Input: part model. Units: mm. Frame: model coordinates. Give positions to 0.01 mm unless a question says otherwise; leave off trailing zeros. Loops run counter-clockwise (first coordinate to the right, second up) from the corner with the lowest first, then second, coordinate; pieces in that order, holes last. Notation, with made-up numbers: (11.25, 80) -> (39.25, 80) arc R33 ccw to (39.25, 113) -> close; hole circle Ø5 at (0, 73). An arc over 180 degrees is marked (long way). Answer as a JSON object with one key per item and string values.
```python
from build123d import *

# Parameters (mm, degrees)
SKETCH_W        = 40
SKETCH_H        = 20
PAD_DEPTH       = 0.8
SKETCH001_R     = 1.7
POCKET_DEPTH    = 90.258029
SKETCH002_W     = 12.04
SKETCH002_H     = 10.6
POCKET001_DEPTH = 0.801


with BuildPart() as part:
    # Sketch → Pad (new body)
    with BuildSketch(Plane.XZ):
        Rectangle(SKETCH_W, SKETCH_H)
    extrude(amount=PAD_DEPTH)

    # Sketch001 (on Face6 of Pad) → Pocket (cut, through all)
    with BuildSketch(Plane.XZ.offset(0.8)):
        with Locations((-15.25, 0)):
            Circle(SKETCH001_R)
    pocket = extrude(amount=-POCKET_DEPTH, mode=Mode.SUBTRACT)

    # Mirrored: Pocket across YZ
    add(pocket.mirror(Plane.YZ), mode=Mode.SUBTRACT)

    # Sketch002 (on Face5 of Mirrored) → Pocket001 (cut, through all)
    with BuildSketch(Plane.XZ.offset(0.8)):
        with Locations((0, 1.445)):
            Rectangle(SKETCH002_W, SKETCH002_H)
    extrude(amount=-POCKET001_DEPTH, mode=Mode.SUBTRACT)


solid = part.part
```
Q1. Ray query, line 1 along Z through (x, y) = (15.25, -0.5); line 2 along Z through (x, y) = (-2, -0.45) (3 decimals); line 3 along X through (y, z) = (-0.55, -2.5). Return the intervals inside material, ascending.
Evaluation:
{"line 1": "z = -10 to -1.7, 1.7 to 10", "line 2": "z = -10 to -3.855, 6.745 to 10", "line 3": "x = -20 to -6.02, 6.02 to 20"}
Q2. Section C-C, the plane x = 2.5. Return the cut outline in (y, z) (3 decimals), then the cut area to 3 significant figures.
Evaluation:
{"outline": "(-0.8, -10) -> (0, -10) -> (0, -3.855) -> (-0.8, -3.855) -> close; (-0.8, 6.745) -> (0, 6.745) -> (0, 10) -> (-0.8, 10) -> close", "area": "7.52 mm2"}
Q3. Draft query along Z for faces 1 (the cylindrical face through (13.63, -0.41, 0.51)), 2 (the flat face through (-0.3, -0.8, -4.3)). Return one class per face: +Z half, -Z half, draft (parallel to the pull), parting line (faces both ways), or undercut.
Evaluation:
{"face 1": "undercut", "face 2": "draft"}
Q4. Pin query (flat end, axial travel): pin 1 (5 mm diameter, centred on x = -10, z = -4, fed in from +Y). Return the tip coordinate at first contact, or that it passes through.
Evaluation:
{"pin 1": "stops at y = 0"}
Q5. Section B-B, the plane z = 0. Return the cut outline in (x, y).
Evaluation:
{"outline": "(-20, -0.8) -> (-16.95, -0.8) -> (-16.95, 0) -> (-20, 0) -> close; (-13.55, -0.8) -> (-6.02, -0.8) -> (-6.02, 0) -> (-13.55, 0) -> close; (6.02, -0.8) -> (13.55, -0.8) -> (13.55, 0) -> (6.02, 0) -> close; (16.95, -0.8) -> (20, -0.8) -> (20, 0) -> (16.95, 0) -> close"}
Q6. Section A-A, the plane x = 15.25. Return the cut outline in (y, z), then the cut area to 3 significant figures.
Evaluation:
{"outline": "(-0.8, -10) -> (0, -10) -> (0, -1.7) -> (-0.8, -1.7) -> close; (-0.8, 1.7) -> (0, 1.7) -> (0, 10) -> (-0.8, 10) -> close", "area": "13.3 mm2"}
